```python
from build123d import *

# Parameters (mm, degrees)
SKETCH_7_R      = 15
EXTRUDE_5_DEPTH = 30
SKETCH_8_R      = 15
EXTRUDE_6_DEPTH = 100
SKETCH_9_R      = 15
EXTRUDE_7_DEPTH = 30


with BuildPart() as part:
    # 草图7 → 凸台-拉伸5 (new, symmetric)
    with BuildSketch(Plane(origin=(0, 0, 0), x_dir=(0, 0, -1), z_dir=(1, 0, 0))):
        with Locations(Location((0, 0, 0), (0, 0, 180))):
            Circle(SKETCH_7_R)
    extrude(amount=EXTRUDE_5_DEPTH, both=True)

    # 草图8 → 凸台-拉伸6 (add)
    with BuildSketch(Plane.XY):
        with Locations(Location((0, 0, 0), (0, 0, 90))):
            Circle(SKETCH_8_R)
    extrude(amount=EXTRUDE_6_DEPTH)

    # 草图9 → 凸台-拉伸7 (add, symmetric)
    with BuildSketch(Plane(origin=(0, 0, 0), x_dir=(0, 0, -1), z_dir=(1, 0, 0))):
        with Locations((-100, 0)):
            Circle(SKETCH_9_R)
    extrude(amount=EXTRUDE_7_DEPTH, both=True)


solid = part.part
```
Input: part model. Units: mm. Frame: model coordinates. A direction names the side the tool comes from. Give positions to 0.01 mm unless a question says otherwise; leave off trailing zeros. Loops run counter-clockwise (first coordinate to the right, second up) from the corner with the lowest first, then second, coordinate; pieces in that order, holes last. Notation, with made-up numbers: (65, 22.5) -> (122, 22.5) arc R22 ccw to (122, 52.5) -> close; hole circle Ø3 at (79, 40). An arc over 180 degrees is marked (long way). Use a Markdown table: item, result.
Q1. Pull-direction query (Z, two-part tool) for faces 1 (the flat face through (30, 0, 100)), 2 (the cylindrical face through (0.42, -0.66, -14.985)); classes: pulls with the +Z half, pulls with the -Z half, needs draft (parallel to the pull), parting line crosses it, or undercut.
Entries:
| item | result |
|---|---|
| face 1 | needs draft |
| face 2 | undercut |
Q2. Section query C-C, the plane z = 47.5. Return the cut outline in (x, y), plus the area to 3 significant figures.
Entries:
| item | result |
|---|---|
| outline | circle Ø30 at (0, 0) |
| area | 707 mm² |
Q3. Ray query, probe 1 along Z at (x, y) = (-26.5, 1); probe 2 along Z at (x, y) = (-17, -11); probe 3 along X at (y, z) = (5, 64.5). Return the intervals inside material, ascending. Write a range as from..to.
Entries:
| item | result |
|---|---|
| probe 1 | z = -14.97..14.97, 85.03..114.97 |
| probe 2 | z = -10.2..10.2, 89.8..110.2 |
| probe 3 | x = -14.14..14.14 |
Q4. Section query B-B, the plane y = -3.75. Return the cut outline in (x, z), plus the area to 3 significant figures.
Entries:
| item | result |
|---|---|
| outline | (-30, -14.52) -> (30, -14.52) -> (30, 14.52) -> (14.52, 14.52) -> (14.52, 85.48) -> (30, 85.48) -> (30, 114.52) -> (-30, 114.52) -> (-30, 85.48) -> (-14.52, 85.48) -> (-14.52, 14.52) -> (-30, 14.52) -> close |
| area | 5,550 mm² |
Q5. First-contact query: P1, Ø4, axis at x = 13, z = 63, coming from the -Y side; P2, Ø10, axis at x = 17.5, z = 72.5, coming from the +Y side; P3, Ø1, axis at x = -20, y = 3.5, coming from the +Z side. Flat tips, straight axial feed; report the tip coordinate or a pass-through.
Entries:
| item | result |
|---|---|
| P1 | stops at y = -10.2 |
| P2 | stops at y = 8.29 |
| P3 | stops at z = 114.7 |
Q6. Access query for faces 3 (the cylindrical face through (-4.506, 14.307, 49.3)), 4 (the flat face through (30, 0, 0)). Directions: +Z, -Z, +X, -X, +Y, -Y. A direction counts if a zero-diameter tool reaches every point of the face in a straight line with its end or side. Return the directions, or none.
Entries:
| item | result |
|---|---|
| face 3 | none |
| face 4 | +Z, -Z, +X, +Y, -Y |
Q7. Section query A-A, the plane x = 22. Return the cut outline in (y, z).
Entries:
| item | result |
|---|---|
| outline | circle Ø30 at (0, 0); circle Ø30 at (0, 100) |
Q8. Section query D-D, the plane z = 105.5. Return the cut outline in (x, y).
Entries:
| item | result |
|---|---|
| outline | (-30, -13.96) -> (30, -13.96) -> (30, 13.96) -> (-30, 13.96) -> close |
